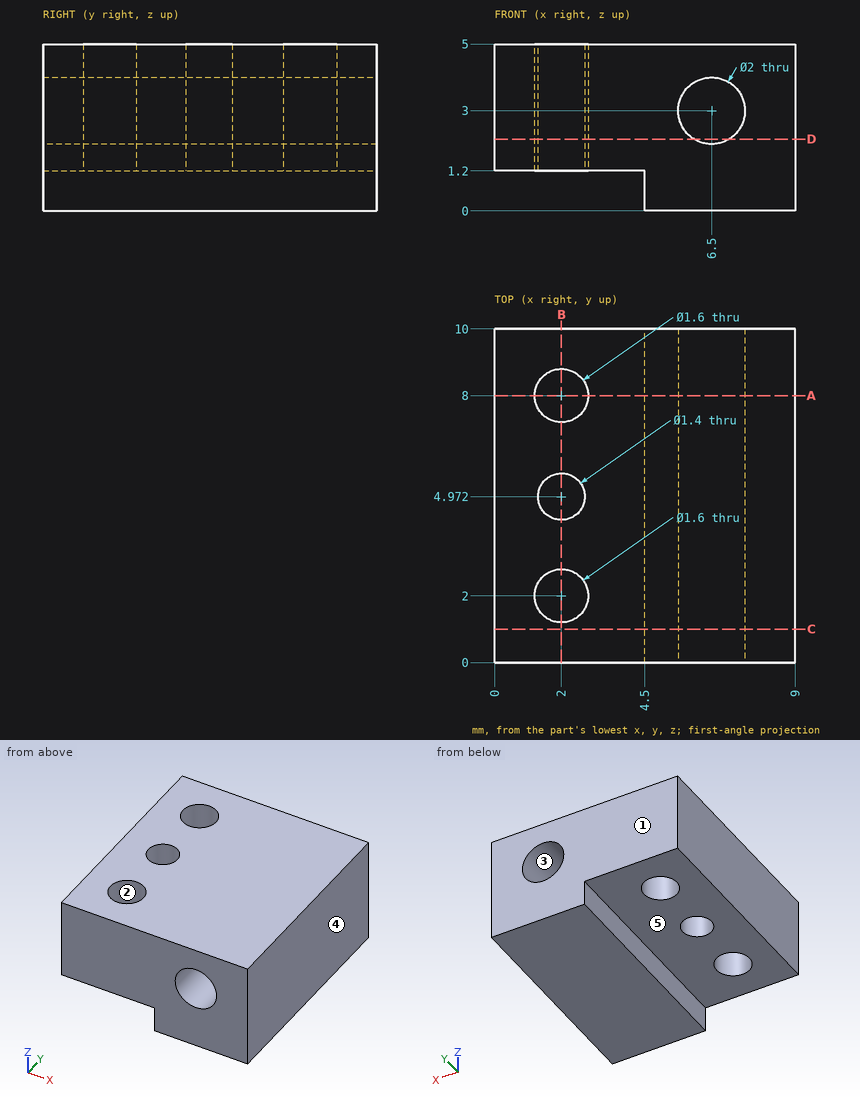
The drawing under review shows one solid part. Ordinate dimensions are in mm from its lowest x, y, z. A direction names the side the tool comes from. Coordinates: 2 decimals unless noted, no trailing zeros. Write each loop counter-clockwise with the first axis right and the second up, starting at its lowest first coordinate (ties: lowest second). Pieces come first, ordered by that corner, then holes.
1) Machinability: for the marked faces 4 and 5, which of the approach directions +Z, -Z, +X, -X, +Y, -Y give a long, thin tool a straight path to every point of the face, cutting with its end or side? Answer none if there is none.
2) Insertion check: pin 1 (5 mm diameter, centred on x = 1.5, y = 5.5, fed in from -Z). The pin has a flat end and moves straight along its axis. Give the tip position at first contact, or say it passes through.
3) Add section C-C (y = 1). Write out the cut boundary in (x, z).
4) To check wall thickness, follow L1, parallel to Y at x = 2, z = 2.05; L2, parallel to X at y = 5.5, z = 3; L3, parallel to X at y = 4.75, z = 3.4. State the ranges of each line that lie inside material, in increasing order.
5) Add section B-B (x = 2). Write out the cut boundary in (y, z).
6) Add section D-D (z = 2.15). Write out the cut boundary in (x, y).
7) Mouldability with a two-part tool opening along Y and no side actions: class the marked faces 1, 2 and 3 as +Y half, -Y half, draft (parallel to the pull), parting line (faces both ways), or undercut.
8) Add section A-A (y = 8). Write out the cut boundary in (x, z).
Check result:
1. face 4: +Z, -Z, +X, +Y, -Y
1. face 5: -Z, -X, +Y, -Y
2. pin 1: stops at z = 1.2
3. outline: (0, 1.2) - (4.5, 1.2) - (4.5, 0) - (9, 0) - (9, 5) - (0, 5) - close; hole circle Ø2 at (6.5, 3)
4. L1: y = 0 to 1.2, 2.8 to 4.27, 5.67 to 7.2, 8.8 to 10
4. L2: x = 0 to 1.54, 2.46 to 5.5, 7.5 to 9
4. L3: x = 0 to 1.34, 2.66 to 5.58, 7.42 to 9
5. outline: (0, 1.2) - (1.2, 1.2) - (1.2, 5) - (0, 5) - close; (2.8, 1.2) - (4.27, 1.2) - (4.27, 5) - (2.8, 5) - close; (5.67, 1.2) - (7.2, 1.2) - (7.2, 5) - (5.67, 5) - close; (8.8, 1.2) - (10, 1.2) - (10, 5) - (8.8, 5) - close
6. outline: (0, 0) - (5.97, 0) - (5.97, 10) - (0, 10) - close; (7.03, 0) - (9, 0) - (9, 10) - (7.03, 10) - close; hole circle Ø1.6 at (2, 2); hole circle Ø1.6 at (2, 8); hole circle Ø1.4 at (2, 4.97)
7. face 1: +Y half
7. face 2: undercut
7. face 3: draft
8. outline: (0, 1.2) - (1.2, 1.2) - (1.2, 5) - (0, 5) - close; (2.8, 1.2) - (4.5, 1.2) - (4.5, 0) - (9, 0) - (9, 5) - (2.8, 5) - close; hole circle Ø2 at (6.5, 3)
